Autodesk Inventor part; units mm, degrees
ref_plane "Work Plane1" through (18, 0, 1) normal (0, 0, -1) x (-1, 0, 0)
ref_plane "Work Plane4" through (0, 0, 18.75) normal (-1, 0, 0) x (0, 0, 1)
ref_plane "YZ Plane" through (0, 0, 0) normal (1, 0, 0) x (0, 1, 0)
sketch "Sketch1" plane through (0, 0, 0) normal (0, 1, 0) x (-1, 0, 0)
  line L0 (18, 22) -> (-18, 22)
  line L1 (-18, 15.5) -> (-16, 15.5)
  line L2 (-16, 15.5) -> (-16, -15.5)
  line L3 (-16, -13.5) -> (-18, -13.5)
  line L4 (-18, -20) -> (18, -20)
  line L5 (18, -13.5) -> (16, -13.5)
  line L6 (16, -15.5) -> (16, 15.5)
  line L7 (16, 15.5) -> (18, 15.5)
  arc A0 (-18, 22) -> (-18, 15.5) centre (-18, 18.75) ccw
  arc A1 (18, 15.5) -> (18, 22) centre (18, 18.75) ccw
  arc A2 (18, -20) -> (18, -13.5) centre (18, -16.75) ccw
  arc A3 (-18, -13.5) -> (-18, -20) centre (-18, -16.75) ccw
  line L8 (16, -15.5) -> (-16, -15.5)
  line L9 (-16, 15.5) -> (16, 15.5)
  circle A4 centre (18, -16.75) radius 1.25
  circle A5 centre (-18, -16.75) radius 1.25
  circle A6 centre (-18, 18.75) radius 1.25
  circle A7 centre (18, 18.75) radius 1.25
  point P0 (0, 0)
  point P1 (-3.7522, -13.5)
  point P2 (0, 22)
  point P3 (0, -20)
  point P4 (16, 0)
  point P5 (-16, 0)
  point P6 (0, -15.5)
  point P7 (0, 15.5)
  point P8 (0, 22)
  point P9 (-16, 0)
  dimension "d0" = 32
  dimension "d1" = 42
  dimension "d2" = 31
  dimension "d4" = 2.5
  dimension "d6" = 2
  dimension "d7" = 2
extrude "Extrusion1" add sketch "Sketch1" against normal blind 1.57
extrude "Extrusion2" add sketch "Sketch1" along normal blind 1 contours L6 L8 L2 L9
ref_plane "Work Plane1" through (18, 0, 1) normal (0, 0, -1) x (-1, 0, 0)
ref_plane "Work Plane4" through (0, 0, 18.75) normal (-1, 0, 0) x (0, 0, 1)
ref_plane "Work Plane2" through (21.25, 0, 18.75) normal (1, 0, 0) x (0, 0, -1)
ref_plane "Work Plane3" through (-21.25, 0, 18.75) normal (-1, 0, 0) x (0, 0, 1)
ref_plane "Plano de trabajo5" through (-21.25, -1.57, 18.75) normal (-1, 0, 0) x (0, 0, 1)
properties part number "Pantalla" material "Steel, Mild, Welded"
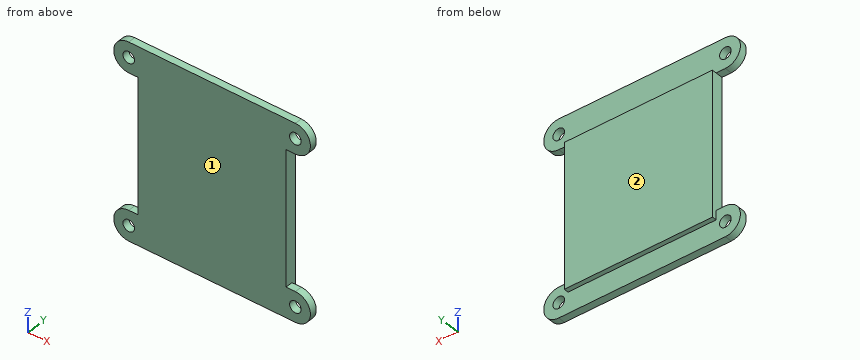
Source: CAD feature listing. Evaluate the final solid. Frame: model axes, mm. Face numbers are marked on the shaded views. Give positions to 0.01 mm unless a question says otherwise; leave off trailing zeros. Loops run counter-clockwise (first coordinate to the right, second up) from the corner with the lowest first, then second, coordinate; pieces in that order, holes last. Notation, with made-up numbers: (49.25, 27.25) -> (85.25, 27.25) arc R10 cw to (85.25, 45.25) -> close; hole circle Ø11 at (24, 29.5). An arc over 180 degrees is marked (long way). Use a Markdown table: item, result. Add a question column.
1) Section query C-C, the plane x = 18.5. Return the cut outline in (y, z).
2) Pull-direction query (Y, two-part tool) for the marked faces 1 and 2; classes: +Y half, -Y half, draft (parallel to the pull), parting line (faces both ways), or undercut.
3) Section query B-B, the plane y = -0.9. Return the cut outline in (x, z), then the cut area to 3 significant figures.
4) Section query A-A, the plane z = 18.75. Return the cut outline in (x, y), then the cut area to 3 significant figures.
5) Section query D-D, the plane x = -14. Return the cut outline in (y, z).
6) First-contact query: pin 1 (1.3 mm diameter, centred on y = -1, z = -2.5, fed in from -X); pin 2 (4 mm diameter, centred on x = -18, z = -16.75, fed in from +Y); pin 3 (1.5 mm diameter, centred on y = -1, z = 13, fed in from +X). Flat tips, straight axial feed; report the tip coordinate or a pass-through.
7) Line query: line 1 along Z through (x, y) = (18, -0.95); line 2 along X through (y, z) = (-0.3, -17); line 3 along Z through (x, y) = (-19, -0.75). Output: solid intervals per line, ascending. Write a range as [from, to].
Numbers:
| question | item | result |
|---|---|---|
| 1 | outline | (-1.57, -19.96) -> (0, -19.96) -> (0, -17.9) -> (-1.57, -17.9) -> close; (-1.57, -15.6) -> (0, -15.6) -> (0, -13.54) -> (-1.57, -13.54) -> close; (-1.57, 15.54) -> (0, 15.54) -> (0, 17.6) -> (-1.57, 17.6) -> close; (-1.57, 19.9) -> (0, 19.9) -> (0, 21.96) -> (-1.57, 21.96) -> close |
| 2 | face 1 | -Y half |
| 2 | face 2 | +Y half |
| 3 | outline | (-18, -20) -> (18, -20) arc R3.25 ccw to (18, -13.5) -> (16, -13.5) -> (16, 15.5) -> (18, 15.5) arc R3.25 ccw to (18, 22) -> (-18, 22) arc R3.25 ccw to (-18, 15.5) -> (-16, 15.5) -> (-16, -13.5) -> (-18, -13.5) arc R3.25 ccw to start; hole circle Ø2.5 at (-18, -16.75); hole circle Ø2.5 at (-18, 18.75); hole circle Ø2.5 at (18, -16.75); hole circle Ø2.5 at (18, 18.75) |
| 3 | area | 1,440 mm2 |
| 4 | outline | (-21.25, -1.57) -> (-19.25, -1.57) -> (-19.25, 0) -> (-21.25, 0) -> close; (-16.75, -1.57) -> (16.75, -1.57) -> (16.75, 0) -> (-16.75, 0) -> close; (19.25, -1.57) -> (21.25, -1.57) -> (21.25, 0) -> (19.25, 0) -> close |
| 4 | area | 58.9 mm2 |
| 5 | outline | (-1.57, -20) -> (0, -20) -> (0, -15.5) -> (1, -15.5) -> (1, 15.5) -> (0, 15.5) -> (0, 22) -> (-1.57, 22) -> close |
| 6 | pin 1 | stops at x = -16 |
| 6 | pin 2 | stops at y = 0 |
| 6 | pin 3 | stops at x = 16 |
| 7 | line 1 | z = [-20, -18], [-15.5, -13.5], [15.5, 17.5], [20, 22] |
| 7 | line 2 | x = [-21.24, -19.22], [-16.78, 16.78], [19.22, 21.24] |
| 7 | line 3 | z = [-19.84, -17.5], [-16, -13.66], [15.66, 18], [19.5, 21.84] |
